```python
from build123d import *

# Parameters (mm, degrees)
F1_DEPTH = 2.54
F3_DEPTH = 2.54
F4_R     = 10.795
F4_R_2   = 1.7
F5_DEPTH = 5.081


with BuildPart() as f1:
    # F0 (on Top) → F1 (new body)
    with BuildSketch(Plane.XY):
        with BuildLine():
            Line((-19.05, -15.875), (19.05, -15.875))
            ThreePointArc((19.05, -15.875), (23.540128, -14.015128), (25.4, -9.525))
            Line((25.4, -9.525), (25.4, 9.525))
            ThreePointArc((25.4, 9.525), (23.540128, 14.015128), (19.05, 15.875))
            Line((19.05, 15.875), (-19.05, 15.875))
            ThreePointArc((-19.05, 15.875), (-23.540128, 14.015128), (-25.4, 9.525))
            Line((-25.4, 9.525), (-25.4, -9.525))
            ThreePointArc((-25.4, -9.525), (-23.540128, -14.015128), (-19.05, -15.875))
        make_face()
    extrude(amount=F1_DEPTH)

    # F2 (on face) → F3 (join)
    with BuildSketch(Plane.XY.offset(2.54)):
        with BuildLine():
            Line((-12.065, -11.811), (12.065, -11.811))
            ThreePointArc((12.065, -11.811), (14.759077, -10.695077), (15.875, -8.001))
            Line((15.875, -8.001), (15.875, 5.037175))
            ThreePointArc((15.875, 5.037175), (15.719597, 5.911989), (15.272403, 6.679756))
            Line((15.272403, 6.679756), (11.682856, 10.913581))
            ThreePointArc((11.682856, 10.913581), (10.813031, 11.575751), (9.745453, 11.811))
            Line((9.745453, 11.811), (-9.745453, 11.811))
            ThreePointArc((-9.745453, 11.811), (-10.813031, 11.575751), (-11.682856, 10.913581))
            Line((-11.682856, 10.913581), (-15.272403, 6.679756))
            ThreePointArc((-15.272403, 6.679756), (-15.719597, 5.911989), (-15.875, 5.037175))
            Line((-15.875, 5.037175), (-15.875, -8.001))
            ThreePointArc((-15.875, -8.001), (-14.759077, -10.695077), (-12.065, -11.811))
        make_face()
    extrude(amount=F3_DEPTH)

    # F4 (on face) → F5 (cut, through all)
    with BuildSketch(Plane.XY.offset(5.08)):
        Circle(F4_R)
        with Locations((-20, 0)):
            Circle(F4_R_2)
        with Locations((20, 0)):
            Circle(F4_R_2)
    extrude(amount=-F5_DEPTH, mode=Mode.SUBTRACT)


solid = f1.part
```
Geometry check sheet. Reference: the model listing, model coordinates, mm. A direction names the side the tool comes from. Coordinates: 2 decimals unless noted, no trailing zeros. Loops run counter-clockwise (first coordinate to the right, second up) from the corner with the lowest first, then second, coordinate; pieces in that order, holes last. Notation, with made-up numbers: (86.5, 55) -> (130.5, 55) arc R20 ccw to (130.5, 61) -> close; hole circle Ø8 at (83, -1). An arc over 180 degrees is marked (long way). Put each result on its own line as item: value.
1) Gauge pin test, flat ends, axial feed: pin 1 Ø2 at (x, z) = (-0.5, 4) entering from -Y; pin 2 Ø0.8 at (y, z) = (-1, 3.5) entering from -X (3 decimals); pin 3 Ø3 at (y, z) = (-3, 4.5) entering from +X (3 decimals). Record the tip position at first contact, or that the pin passes through.
Result set:
pin 1: stops at y = -11.81
pin 2: stops at x = -15.875
pin 3: stops at x = 15.875
2) Thickness scan on line 1 (Y direction, x = 0, z = 1.25) (3 decimals); line 2 (Y direction, x = 0, z = 4.05) (3 decimals); line 3 (Z direction, x = -17.5, y = -9.5). Record the ranges inside material, lowest first.
Result set:
line 1: y = -15.875 to -10.795, 10.795 to 15.875
line 2: y = -11.811 to -10.795, 10.795 to 11.811
line 3: z = 0 to 2.54
3) Cross-section at C-C on z = 1.4. Record the boundary of the cut face in (x, y) (3 decimals).
Result set:
outline: (-25.4, -9.525) arc R6.35 ccw to (-19.05, -15.875) -> (19.05, -15.875) arc R6.35 ccw to (25.4, -9.525) -> (25.4, 9.525) arc R6.35 ccw to (19.05, 15.875) -> (-19.05, 15.875) arc R6.35 ccw to (-25.4, 9.525) -> close; hole circle Ø3.4 at (-20, 0); hole circle Ø21.59 at (0, 0); hole circle Ø3.4 at (20, 0)
4) Tool access check on faces 4 (the cylindrical face through (10.83, 11.57, 3.79)), 5 (the cylindrical face through (-15.715, 5.924, 3.792)), 6 (the cylindrical face through (-14.789, -10.665, 3.792)). Record the directions out of +Z, -Z, +X, -X, +Y, -Y that give a thin tool (end or side, any length) a straight path to the whole face; none if there is none.
Result set:
face 4: +Z, +X, +Y
face 5: +Z, -X, +Y
face 6: +Z, -X, -Y
5) Release check for a two-part mould opening along Y. For faces 1 (the cylindrical face through (21.57, -0.65, 1.29)), 2 (the flat face through (0, -11.811, 4)), 3 (the cylindrical face through (23.589, 13.965, 1.252)) record: released by +Y, released by -Y, zero draft, split by the parting line, or undercut.
Result set:
face 1: undercut
face 2: released by -Y
face 3: released by +Y
6) Cross-section at D-D on y = 9. Record the boundary of the cut face in (x, z), plus the area to 3 significant figures.
Result set:
outline: (-25.4, 0) -> (-5.96, 0) -> (-5.96, 5.08) -> (-13.31, 5.08) -> (-13.31, 2.54) -> (-25.4, 2.54) -> close; (5.96, 0) -> (25.4, 0) -> (25.4, 2.54) -> (13.31, 2.54) -> (13.31, 5.08) -> (5.96, 5.08) -> close
area: 136 mm^2
7) Cross-section at A-A on y = 0. Record the boundary of the cut face in (x, z) (3 decimals), plus the area to 3 significant figures.
Result set:
outline: (-25.4, 0) -> (-21.7, 0) -> (-21.7, 2.54) -> (-25.4, 2.54) -> close; (-18.3, 0) -> (-10.795, 0) -> (-10.795, 5.08) -> (-15.875, 5.08) -> (-15.875, 2.54) -> (-18.3, 2.54) -> close; (10.795, 0) -> (18.3, 0) -> (18.3, 2.54) -> (15.875, 2.54) -> (15.875, 5.08) -> (10.795, 5.08) -> close; (21.7, 0) -> (25.4, 0) -> (25.4, 2.54) -> (21.7, 2.54) -> close
area: 82.7 mm^2
8) Cross-section at B-B on x = 0. Record the boundary of the cut face in (y, z) (3 decimals).
Result set:
outline: (-15.875, 0) -> (-10.795, 0) -> (-10.795, 5.08) -> (-11.811, 5.08) -> (-11.811, 2.54) -> (-15.875, 2.54) -> close; (10.795, 0) -> (15.875, 0) -> (15.875, 2.54) -> (11.811, 2.54) -> (11.811, 5.08) -> (10.795, 5.08) -> close
